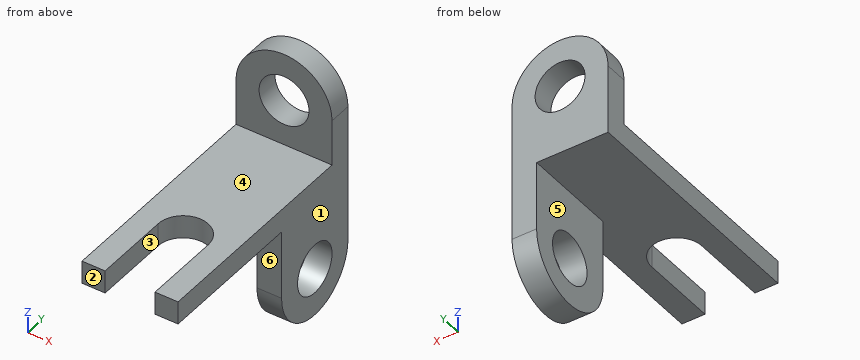
```python
from build123d import *

# Parameters (mm, degrees)
F1_DEPTH = 6
F3_DEPTH = 6
F5_DEPTH = 6.4


with BuildPart() as f1:
    # F0 (on Top) → F1 (new body)
    with BuildSketch(Plane.XY):
        with BuildLine():
            Line((12.5, -32), (12.5, 32))
            Line((12.5, 32), (-12.5, 32))
            Line((-12.5, 32), (-12.5, -32))
            Line((-12.5, -32), (-6.5, -32))
            Line((-6.5, -32), (-6.5, -12))
            ThreePointArc((-6.5, -12), (0, -5.5), (6.5, -12))
            Line((6.5, -12), (6.5, -32))
            Line((6.5, -32), (12.5, -32))
        make_face()
    extrude(amount=F1_DEPTH)

    # F2 (on face) → F3 (join)
    with BuildSketch(Plane(origin=(0, 32, 0), x_dir=(-1, 0, 0), z_dir=(0, 1, 0))):
        with BuildLine():
            Line((-12.5, 18), (-12.5, 6))
            Line((-12.5, 6), (12.5, 6))
            Line((12.5, 6), (12.5, 18))
            Line((12.5, 18), (6.5, 18))
            ThreePointArc((6.5, 18), (0, 11.5), (-6.5, 18))
            Line((-6.5, 18), (-12.5, 18))
        make_face()
        with BuildLine():
            ThreePointArc((12.5, 18), (0, 30.5), (-12.5, 18))
            Line((-12.5, 18), (-6.5, 18))
            ThreePointArc((-6.5, 18), (0, 24.5), (6.5, 18))
            Line((6.5, 18), (12.5, 18))
        make_face()
    extrude(amount=-F3_DEPTH)

    # F4 (on face) → F5 (join)
    with BuildSketch(Plane.YZ.offset(12.5)):
        with BuildLine():
            Line((32, -18), (32, 0))
            Line((32, 0), (7, 0))
            Line((7, 0), (7, -18))
            Line((7, -18), (13, -18))
            ThreePointArc((13, -18), (19.5, -11.5), (26, -18))
            Line((26, -18), (32, -18))
        make_face()
        with BuildLine():
            ThreePointArc((7, -18), (19.5, -30.5), (32, -18))
            Line((32, -18), (26, -18))
            ThreePointArc((26, -18), (19.5, -24.5), (13, -18))
            Line((13, -18), (7, -18))
        make_face()
    extrude(amount=-F5_DEPTH)


solid = f1.part
```
Part model, mm, in its own coordinate system. Face numbers are marked on the shaded views. A direction names the side the tool comes from. Round coordinates to 2 decimals unless told otherwise and drop trailing zeros. Write each loop counter-clockwise with the first axis right and the second up, starting at its lowest first coordinate (ties: lowest second). Pieces come first, ordered by that corner, then holes. Notation, with made-up numbers: (9, 6.25) -> (46, 6.25) arc R26 cw to (46, 29.25) -> close; hole circle Ø3 at (81, 62.25). An arc over 180 degrees is marked (long way). Return JSON: item names as keys, results as strings. Group by question number.
Q1. Pin check, flat tips, straight feed: pin 1 (21 mm diameter, centred on y = 19.5, z = -18, fed in from -X); pin 2 (12.5 mm diameter, centred on x = 3.5, y = -12, fed in from -Z); pin 3 (7.5 mm diameter, centred on x = 6, y = 5, fed in from +Z). Stop position of each tip, or through.
Q2. Saw through at A-A on x = 0. Write the cut outline in (y, z).
Q3. Which spindle directions (+Z, -Z, +X, -X, +Y, -Y) get a long thin tool onto all of the face, cutting with end or side? Do the marked faces 4, 5 and 6. Say none if no direction does.
Q4. Saw through at D-D on x = 9.5. Write the cut outline in (y, z), plus the area to 3 significant figures.
Q5. Saw through at C-C on z = 1. Write the cut outline in (x, y), plus the area to 3 significant figures.
Q6. Mould opens along X. For the marked faces 1, 2 and 3 say: pulls with the +X half, pulls with the -X half, needs draft (parallel to the pull), parting line crosses it, or undercut.
Q7. Saw through at B-B on y = -24. Write the cut outline in (x, z).
Q8. Probe L1, parallel to Z at x = 10.75, y = 19.5; L2, parallel to Y at x = 9, z = -18; L3, parallel to Z at x = 0, y = 28. List the from-to ranges inside material, lowest first. Write a range as [from, to].
Answer:
{
 "1": {"pin 1": "x = 6.1", "pin 2": "z = 0", "pin 3": "z = 6"},
 "2": {"outline": "(-5.5, 0) -> (32, 0) -> (32, 11.5) -> (26, 11.5) -> (26, 6) -> (-5.5, 6) -> close; (26, 24.5) -> (32, 24.5) -> (32, 30.5) -> (26, 30.5) -> close"},
 "3": {"face 4": "+Z, +X, -X, -Y", "face 5": "-Z, -X, +Y, -Y", "face 6": "-Z, +X, -X, -Y"},
 "4": {"outline": "(-32, 0) -> (7, 0) -> (7, -18) arc R12.5 ccw to (32, -18) -> (32, 26.12) -> (26, 26.12) -> (26, 6) -> (-32, 6) -> close; hole circle Ø13 at (19.5, -18)", "area": "1,070 mm2"},
 "5": {"outline": "(-12.5, -32) -> (-6.5, -32) -> (-6.5, -12) arc R6.5 cw to (6.5, -12) -> (6.5, -32) -> (12.5, -32) -> (12.5, 32) -> (-12.5, 32) -> close", "area": "1,270 mm2"},
 "6": {"face 1": "pulls with the +X half", "face 2": "needs draft", "face 3": "undercut"},
 "7": {"outline": "(-12.5, 0) -> (-6.5, 0) -> (-6.5, 6) -> (-12.5, 6) -> close; (6.5, 0) -> (12.5, 0) -> (12.5, 6) -> (6.5, 6) -> close"},
 "8": {"L1": "[-30.5, -24.5], [-11.5, 6]", "L2": "[7, 13], [26, 32]", "L3": "[0, 11.5], [24.5, 30.5]"}
}
